Could you check a few things on this drawing? It's one solid part, dimensions in mm from its lowest x, y, z. A direction names the side the tool comes from. Give positions to 0.01 mm unless a question says otherwise; leave off trailing zeros. Order: outer loops, then holes, each group sorted by start corner. A loop starts at its lowest first (then second) coordinate and runs counter-clockwise, first axis right, second up.
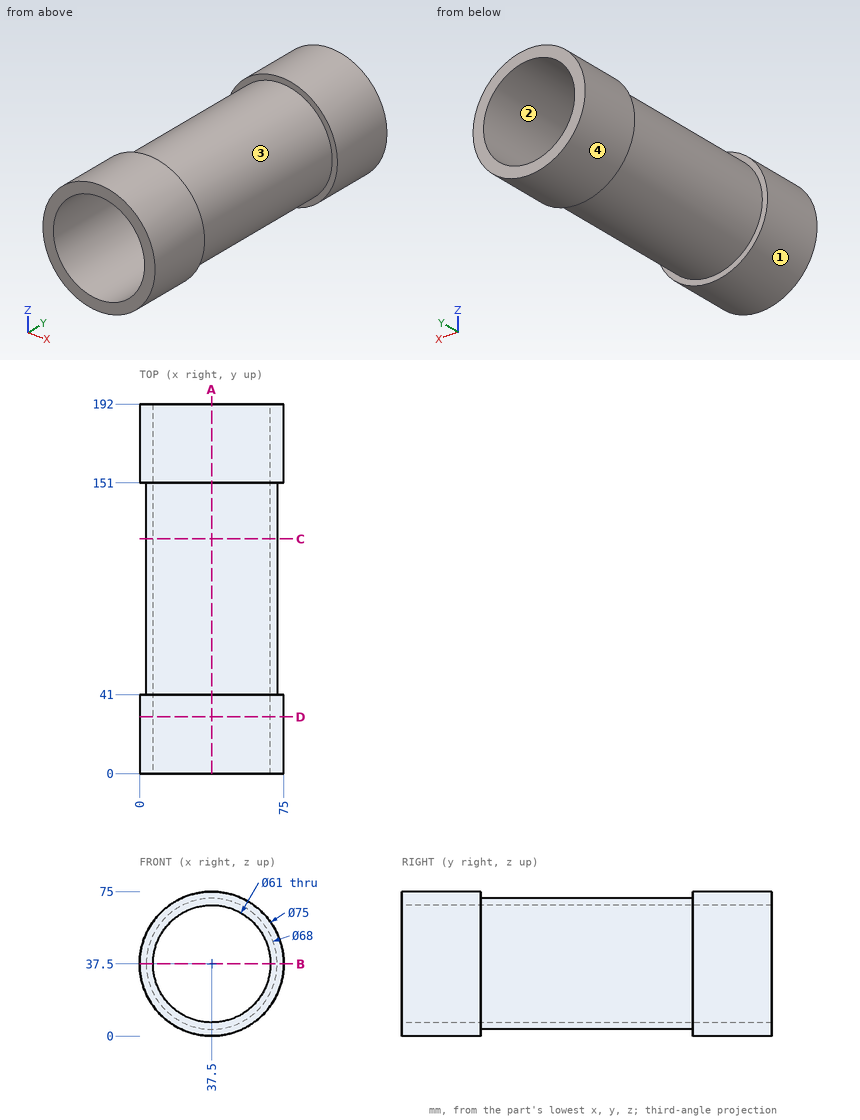
Q1. If we section it at D-D on y = 29.5: List the corners of the cut face in (x, z) for me.
Filled sheet:
outline: circle Ø75 at (37.5, 37.5); hole circle Ø61 at (37.5, 37.5)
Q2. I need wall thicknesses on L1, parallel to X at y = 44, z = 37; L2, parallel to Y at x = 4, z = 51. Which ranges of each line are inside material? Lowest first, please.
Filled sheet:
L1: x = 3.5 to 7, 68 to 71.5
L2: y = 0 to 41, 151 to 192
Q3. If we section it at B-B on z = 37.5: List the corners of the cut face in (x, y) for me.
Filled sheet:
outline: (0, 0) - (7, 0) - (7, 192) - (0, 192) - (0, 151) - (3.5, 151) - (3.5, 41) - (0, 41) - close; (68, 0) - (75, 0) - (75, 41) - (71.5, 41) - (71.5, 151) - (75, 151) - (75, 192) - (68, 192) - close
Q4. If we section it at C-C on y = 122: List the corners of the cut face in (x, z) for me, plus the area to 3 significant figures.
Filled sheet:
outline: circle Ø68 at (37.5, 37.5); hole circle Ø61 at (37.5, 37.5)
area: 709 mm2
Q5. I'm going to push flat-ended pins straight in: P1, Ø10, axis at x = 40, y = 168, coming from the -Z side; P2, Ø10, axis at y = 27.5, z = 19, coming from the -X side; P3, Ø1.5, axis at x = 49.5, y = 42, coming from the +Z side. Where does each tip first touch, or does it pass through?
Filled sheet:
P1: stops at z = 0
P2: stops at x = 2.51
P3: stops at z = 69.58
Q6. Thinking about a two-plate mould opening in X: for the marked faces 1 and 2, which applies, released by +X, released by -X, zero draft, split by the parting line, or undercut?
Filled sheet:
face 1: split by the parting line
face 2: undercut
Q7. For the marked faces 3 and 4, which set-ups out of +Z, -Z, +X, -X, +Y, -Y let a thin tool reach every point of the face, with its end or its side?
Filled sheet:
face 3: none
face 4: +Y, -Y
Q8. If we section it at A-A on x = 37.5: List the corners of the cut face in (y, z) for me, plus the area to 3 significant figures.
Filled sheet:
outline: (0, 0) - (41, 0) - (41, 3.5) - (151, 3.5) - (151, 0) - (192, 0) - (192, 7) - (0, 7) - close; (0, 68) - (192, 68) - (192, 75) - (151, 75) - (151, 71.5) - (41, 71.5) - (41, 75) - (0, 75) - close
area: 1,920 mm2
